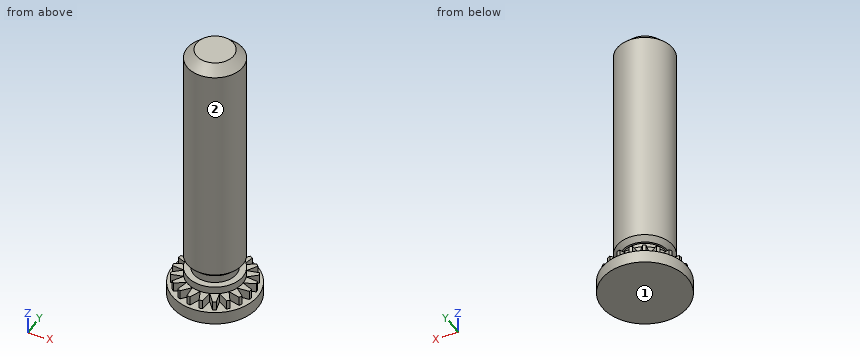
```python
from build123d import *

# Parameters (mm, degrees)
SKETCH_1_R               = 2.3
EXTRUDE_1_DEPTH          = 1.2
SKETCH_2_R               = 1.4999999999999996
EXTRUDE_2_DEPTH          = 1.5
CUT_EXTRUDE_1_DEPTH      = 0.5
PATTERN_CIRCULAR_1_COUNT = 20
SKETCH_4_W               = 0.3500000000000001
SKETCH_4_H               = 0.49999999999999956
SKETCH_6_W               = 12.300000000000002
SKETCH_6_H               = 1.5
CHAMFER_2_SIZE           = 0.5
CUT_EXTRUDE_START        = -0.5
SKETCH_7_R               = 2.3
SKETCH_7_R_2             = 2.1
CUT_EXTRUDE_2_DEPTH      = 0.5


with BuildPart() as part:
    # Эскиз1 → Вытянуть1 (new body)
    with BuildSketch(Plane.XY):
        Circle(SKETCH_1_R)
    extrude(amount=EXTRUDE_1_DEPTH)

    # Эскиз2 → Вытянуть2 (add)
    with BuildSketch(Plane.XY.offset(1.2)):
        Circle(SKETCH_2_R)
    extrude(amount=EXTRUDE_2_DEPTH)

    # Эскиз3 → Вырез-Вытянуть1 (cut)
    with BuildSketch(Plane.XY.offset(1.2)):
        Polygon((-0.33137084989847343, 2.3), (0.33137084989847343, 2.3), (0, 1.4999999999999996), align=None)
    cut_extrude_1 = extrude(amount=-CUT_EXTRUDE_1_DEPTH, mode=Mode.SUBTRACT)

    # Круговой массив1: Вырез-Вытянуть1 ×20 about axis
    pattern_circular_1_axis = Axis((0, -4e-17, 0), (0, 0, 1))
    for i in range(1, PATTERN_CIRCULAR_1_COUNT):
        add(cut_extrude_1.rotate(pattern_circular_1_axis, i * 360 / PATTERN_CIRCULAR_1_COUNT), mode=Mode.SUBTRACT)

    # Эскиз4 → Вырез-Повернуть1 (revolve, cut)
    with BuildSketch(Plane(origin=(0, 0, 0), x_dir=(1, 0, 0), z_dir=(0, 1, 0))):
        with Locations((1.325, -1.8500000000000003)):
            Rectangle(SKETCH_4_W, SKETCH_4_H)
    revolve(axis=Axis((0, 0, 10.642619982654564), (0, 0, -1)), mode=Mode.SUBTRACT)

    # Эскиз6 → Повернуть1 (revolve)
    with BuildSketch(Plane(origin=(0, 0, 0), x_dir=(0, 0, -1), z_dir=(1, 0, 0)), mode=Mode.PRIVATE) as revolve_1_sk:
        with Locations((-8.850000000000001, -0.75)):
            Rectangle(SKETCH_6_W, SKETCH_6_H)
    revolve(revolve_1_sk.sketch.rotate(Axis((0, 0, 2.6999999999999997), (0, 0, 1)), 278.047567557), axis=Axis((0, 0, 2.6999999999999997), (0, 0, 1)))

    # Фаска2
    # the kernel refuses this chamfer: 0.5 mm, written as the material it takes off along each edge
    with BuildSketch(Plane(origin=(0, 0, 15.000000000000002), x_dir=(-0.9901521845161062, -0.1399951838385265, 0), z_dir=(-0.1399951838385265, 0.9901521845161062, 0))) as chamfer_2_piece_1:
        Polygon((1.4999999999999996, -CHAMFER_2_SIZE), (1.5000000000000004 - CHAMFER_2_SIZE, -1.78e-15), (1.5000000000000004, 0), align=None)
    revolve(axis=Axis((0, 0, 15.000000000000002), (0, 0, 1)), mode=Mode.SUBTRACT)

    # Эскиз7 → Вырез-Вытянуть2 (cut)
    with BuildSketch(Plane.XY.offset(1.2).offset(CUT_EXTRUDE_START)):
        with Locations(Location((0, 0, 0), (0, 0, 180))):
            Circle(SKETCH_7_R)
        Circle(SKETCH_7_R_2, mode=Mode.SUBTRACT)
    extrude(amount=CUT_EXTRUDE_2_DEPTH, mode=Mode.SUBTRACT)

    # Фаска3
    # the kernel refuses this chamfer: 0.25 mm, written as the material it takes off along each edge
    with BuildSketch(Plane(origin=(0, 0, 2.0999999999999996), x_dir=(1, 0, 0), z_dir=(0, 1, 0))) as chamfer_3_piece_1:
        with BuildLine():
            Line((1.2429289321881345, 0.00707106781186528), (1.507071067811865, -0.2570710678118653))
            Line((1.507071067811865, -0.2570710678118653), (1.512071067811865, -0.2570710678118653))
            ThreePointArc((1.512071067811865, -0.2570710678118653), (1.5049999999999994, -0.12853553390593264), (1.505, 0))
            Line((1.505, 0), (1.5, 0.00499999999999989))
            ThreePointArc((1.5, 0.00499999999999989), (1.3714644660940674, 0.00499999999999989), (1.2429289321881345, 0.01207106781186518))
            Line((1.2429289321881345, 0.01207106781186518), (1.2429289321881345, 0.00707106781186528))
        make_face()
    revolve(axis=Axis((0, 0, 2.0999999999999996), (0, 0, -1)), mode=Mode.SUBTRACT)


solid = part.part
```
Here's how the part is built. I have some questions about the finished solid (model axes, mm). Face numbers are marked on the shaded views. A direction names the side the tool comes from. Give positions to 0.01 mm unless a question says otherwise; leave off trailing zeros. Write each loop counter-clockwise with the first axis right and the second up, starting at its lowest first coordinate (ties: lowest second). Pieces come first, ordered by that corner, then holes.
(1) If I drill on L1, parallel to Y at x = -0.05, z = 12; L2, parallel to Y at x = -0.45, z = 1.5; L3, parallel to Z at x = 1.95, y = -0.6, over which ranges is the centre line in solid material (lowest first)?
Output values:
L1: y = -1.5 to 1.5
L2: y = -1.43 to 1.43
L3: z = 0 to 0.7
(2) Imagine slicing it at A-A, the plane z = 4. Write out the boundary of the cut face in (x, y), and give its area (3 significant figures).
Output values:
outline: circle Ø3 at (0, 0)
area: 7.07 mm2
(3) On a 3-axis mill with a long thin cutter (end or side, diameter ignored), from which of +Z, -Z, +X, -X, +Y, -Y can I reach the whole of each face in a straight line? I mean the marked faces 1 and 2. Say none if no direction works.
Output values:
face 1: -Z, +X, -X, +Y, -Y
face 2: +Z
(4) Will these pins go through, and if not, where does the flat tip stop? pin 1 (0.5 mm diameter, centred on x = -1, y = 1, fed in from +Z); pin 2 (1 mm diameter, centred on x = -1, z = 13.5, fed in from -Y); pin 3 (1.5 mm diameter, centred on y = 1, z = 12, fed in from +X).
Output values:
pin 1: stops at z = 14.84
pin 2: stops at y = -1.41
pin 3: stops at x = 1.48
